Autodesk Inventor part; units mm, degrees
ref_plane "Work Plane1" through (0, 0, -12) normal (0, 0, 1) x (1, 0, 0)
ref_plane "YZ Plane" through (0, 0, 0) normal (1, 0, 0) x (0, 1, 0)
ref_plane "XZ Plane" through (0, 0, 0) normal (0, 1, 0) x (-1, 0, 0)
sketch "Sketch1" plane through (0, 0, 0) normal (0, 0, 1) x (1, 0, 0)
  line L0 (-199, 163) -> (199, 163)
  line L1 (199, 163) -> (199, -163)
  line L2 (199, -163) -> (-199, -163)
  line L3 (-199, -163) -> (-199, 163)
  line L4 (-199, 163) -> (199, -163) construction
  line L5 (199, 163) -> (-199, -163) construction
  point P0 (0, 0)
  dimension "d0" = 398
  dimension "d1" = 326
extrude "Extrusion1" add sketch "Sketch1" against normal blind 21
ref_plane "Work Plane1" through (0, 0, -12) normal (0, 0, 1) x (1, 0, 0)
sketch "Sketch2" plane through (0, 0, -12) normal (0, 0, 1) x (1, 0, 0)
  line L0 (-206, 163) -> (206, 163) construction
  line L1 (206, -170) -> (-206, -170) construction
  line L2 (-206, -170) -> (-206, 163) construction
  line L3 (-206, 163) -> (206, -170) construction
  line L4 (206, 163) -> (-206, -170) construction
  line L5 (-199, -163) -> (199, -163) construction
  line L6 (-199, 163) -> (-199, -163) construction
  line L7 (199, 163) -> (-199, 163) construction
  line L8 (-199, -163) -> (-199, 163)
  line L9 (199, 10.5) -> (206, 10.5)
  line L10 (206, 10.5) -> (206, -10.5)
  line L11 (206, -10.5) -> (199, -10.5)
  line L12 (199, -10.5) -> (199, 10.5)
  line L13 (199, 10.5) -> (206, -10.5) construction
  line L14 (206, 10.5) -> (199, -10.5) construction
  line L15 (206, -134.9) -> (199, -134.9)
  line L16 (199, -134.9) -> (199, -154.9)
  line L17 (199, -154.9) -> (206, -154.9)
  line L18 (206, -154.9) -> (206, -134.9)
  line L19 (199, -163) -> (-199, -163)
  line L20 (-8, -163) -> (8, -163)
  line L21 (8, -163) -> (8, -170)
  line L22 (8, -170) -> (-8, -170)
  line L23 (-8, -170) -> (-8, -163)
  line L24 (-139, -163) -> (-119, -163)
  line L25 (-119, -163) -> (-119, -170)
  line L26 (-119, -170) -> (-139, -170)
  line L27 (-139, -170) -> (-139, -163)
  line L28 (119, -163) -> (139, -163)
  line L29 (139, -163) -> (139, -170)
  line L30 (139, -170) -> (119, -170)
  line L31 (119, -170) -> (119, -163)
  line L32 (206, 163) -> (206, -170) construction
  line L33 (199, -163) -> (199, 163)
  line L34 (-288.4, 0) -> (288.4, 0)
  line L35 (0, 229.6) -> (0, -236.6)
  line L36 (206, 134.9) -> (199, 134.9)
  line L37 (199, 134.9) -> (199, 154.9)
  line L38 (199, 154.9) -> (206, 154.9)
  line L39 (206, 154.9) -> (206, 134.9)
  line L40 (-199, 10.5) -> (-206, 10.5)
  line L41 (-206, 10.5) -> (-206, -10.5)
  line L42 (-206, -10.5) -> (-199, -10.5)
  line L43 (-199, -10.5) -> (-199, 10.5)
  line L44 (-199, 10.5) -> (-206, -10.5) construction
  line L45 (-206, 10.5) -> (-199, -10.5) construction
  line L46 (-206, -134.9) -> (-199, -134.9)
  line L47 (-199, -134.9) -> (-199, -154.9)
  line L48 (-199, -154.9) -> (-206, -154.9)
  line L49 (-206, -154.9) -> (-206, -134.9)
  line L50 (-199, 134.9) -> (-199, 154.9)
  line L51 (-206, 134.9) -> (-199, 134.9)
  line L52 (-206, 154.9) -> (-206, 134.9)
  line L53 (-199, 154.9) -> (-206, 154.9)
  point P0 (0, 0)
  point P1 (0, -3.5)
  point P2 (202.5, 0)
  point P3 (202.5, 0)
  point P4 (-202.5, 0)
  point P5 (-202.5, 0)
  point P6 (0, -170)
  dimension "d6" = 7
  dimension "d7" = 7
  dimension "d8" = 0
  dimension "d9" = 21
  dimension "d10" = 20
  dimension "d11" = 124.4
  dimension "d12" = 7
  dimension "d13" = 16
  dimension "d14" = 111
  dimension "d15" = 20
  dimension "d16" = 111
  dimension "d17" = 20
extrude "Extrusion2" add sketch "Sketch2" against normal blind 1 contours L51 L52 L53 L8 | L33 L38 L39 L36 | L48 L49 L46 L8 | L19 L25 L26 L27 | L42 L41 L34 L8 | L19 L35 L22 L23 | L34 L41 L40 L8 | L19 L21 L22 L35 | L34 L10 L11 L12 | L12 L9 L10 L34 | L19 L29 L30 L31 | L15 L18 L17 L16
sketch "Sketch3" plane through (0, 0, -12) normal (0, 0, 1) x (1, 0, 0)
  line L0 (-119, -170) -> (-119, -163)
  line L1 (8, -170) -> (8, -163)
  line L2 (119, -163) -> (119, -170)
  point P0 (0, 0)
  point P1 (-202.5, 0)
  point P2 (202.5, 0)
  point P3 (129, -166.5)
  point P4 (0, -166.5)
  point P5 (-129, -166.5)
  point P6 (-119, -166.5)
  point P7 (8, -166.5)
  point P8 (119, -166.5)
hole "Hole1" at (-202.5, 0, -12) at (202.5, 0, -12) at (129, -166.5, -12) at (0, -166.5, -12) at (-129, -166.5, -12) direction (0, 0, -1) diameter 4 end through all
sketch "Sketch4" plane through (0, 0, -12) normal (0, 0, 1) x (1, 0, 0)
  line L0 (206, -134.9) -> (199, -134.9)
  point P0 (0, 0)
  point P1 (202.5, -139.9)
  dimension "d27" = 5
hole "Hole2" at (202.5, -139.9, -12) direction (0, 0, -1) diameter 4 end through all
sketch "Sketch5" plane through (0, 0, -12) normal (0, 0, 1) x (1, 0, 0)
  line L0 (199, -154.9) -> (206, -154.9)
  point P0 (0, 0)
  point P1 (202.5, -148.4)
  point P2 (202.5, -154.9)
  dimension "d35" = 6.5
hole "Hole3" at (202.5, -148.4, -12) direction (0, 0, -1) diameter 6 end through all
mirror "Mirror1" about plane through (0, 0, 0) normal (0, 1, 0) of "Hole2", "Hole3"
mirror "Mirror2" about plane through (0, 0, 0) normal (1, 0, 0) of "Hole2", "Hole3", "Mirror1"
sketch "Sketch6" plane through (0, 0, 0) normal (0, 0, 1) x (1, 0, 0)
  line L0 (-199, -163) -> (199, -163)
  line L1 (199, -163) -> (199, 163)
  line L2 (199, 163) -> (-199, 163)
  line L3 (-199, 163) -> (-199, -163)
  line L4 (-189.5, 153.5) -> (189.5, 153.5)
  line L5 (189.5, 153.5) -> (189.5, -153.5)
  line L6 (189.5, -153.5) -> (-189.5, -153.5)
  line L7 (-189.5, -153.5) -> (-189.5, 153.5)
  point P0 (0, 0)
  dimension "d43" = 9.5
extrude "Extrusion3" cut sketch "Sketch6" against normal blind 1 contours L4 L5 L6 L7
sketch "Sketch7" plane through (0, 0, -21) normal (0, 0, -1) x (-1, 0, 0)
  line L0 (32, 57) -> (127, 57)
  line L1 (127, 57) -> (127, -73)
  line L2 (127, -73) -> (32, -73)
  line L3 (32, -73) -> (32, 57)
  line L4 (199, -163) -> (199, 163)
  line L5 (-199, -163) -> (199, -163)
  point P0 (0, 0)
  dimension "d46" = 72
  dimension "d47" = 90
  dimension "d48" = 95
  dimension "d49" = 130
extrude "Extrusion4" add sketch "Sketch7" along normal blind 30
sketch "Sketch8" plane through (0, 0, -21) normal (0, 0, -1) x (-1, 0, 0)
  line L0 (-159, 91) -> (6, 91)
  line L1 (6, 91) -> (6, -71)
  line L2 (6, -71) -> (-159, -71)
  line L3 (-159, -71) -> (-159, 91)
  line L4 (-199, -163) -> (199, -163)
  line L5 (-199, 163) -> (-199, -163)
  point P0 (0, 0)
  dimension "d52" = 92
  dimension "d53" = 40
  dimension "d54" = 165
  dimension "d55" = 162
extrude "Extrusion5" add sketch "Sketch8" along normal blind 35
sketch "Sketch9" plane through (-6, -71, -21) normal (0, -1, 0) x (1, 0, 0)
  line L0 (0, 0) -> (165, 0)
  line L1 (0, 0) -> (0, -35)
  line L2 (165, -35) -> (0, -35)
  line L3 (165, 0) -> (165, -35)
  line L4 (165, 0) -> (165, -35)
  line L5 (165, -12) -> (135, -35)
  line L6 (165, -35) -> (0, -35)
  point P0 (6, 21)
  dimension "d58" = 23
  dimension "d59" = 30
extrude "Extrusion6" cut sketch "Sketch9" against normal through all contours L3 L2 L5
sketch "Sketch10" plane through (-127, -73, -21) normal (0, -1, 0) x (1, 0, 0)
  line L0 (0, 0) -> (95, 0)
  line L1 (0, 0) -> (0, -30)
  line L2 (95, -30) -> (0, -30)
  line L3 (95, 0) -> (95, -30)
  line L4 (95, -30) -> (0, -30)
  line L5 (12, -30) -> (6, -28)
  line L6 (6, -28) -> (0, -22)
  line L7 (0, 0) -> (0, -30)
  point P0 (127, 21)
  point P1 (0, -22)
  dimension "d62" = 6
  dimension "d63" = 12
  dimension "d64" = 2
  dimension "d65" = 8
extrude "Extrusion7" cut sketch "Sketch10" against normal through all contours L6 L5 L2 L1
properties part number "skærm"
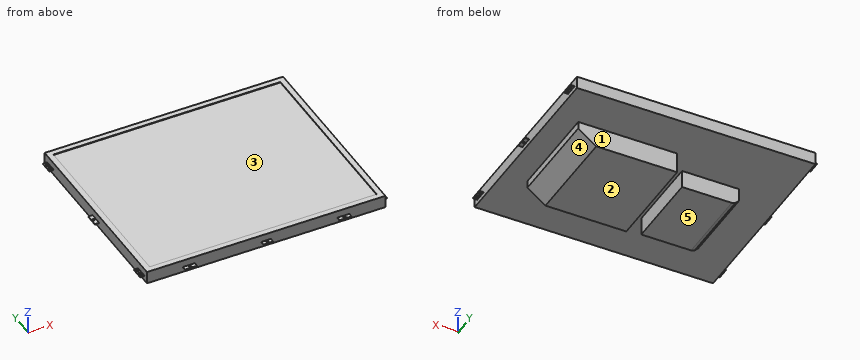
Work out the finished part from the listing and answer in its coordinate system (mm). Face numbers are marked on the shaded views. A direction names the side the tool comes from. Give positions to 0.01 mm unless a question says otherwise; leave off trailing zeros. Loops run counter-clockwise (first coordinate to the right, second up) from the corner with the lowest first, then second, coordinate; pieces in that order, holes last. Notation, with made-up numbers: (57, 1.5) -> (83, 1.5) arc R13 ccw to (83, 26.5) -> close; hole circle Ø6 at (60, -17). An arc over 180 degrees is marked (long way). Put each result on its own line as item: value. Start each with the question number.
Item 1: Each of these flat-tipped pins is pushed along its axis until it touches: P1, Ø4, axis at y = -42, z = -7, coming from the +X side; P2, Ø6.5, axis at x = -202.5, y = 139.9, coming from the +Z side; P3, Ø3, axis at x = 0, y = -166.5, coming from the -Z side; P4, Ø1.1, axis at x = 203.5, z = -12.5, coming from the +Y side. Where does it stop, or does it pass through?
Item 2: The part is cut by section A-A (z = -28). Give the vertices of the cut face in (x, y).
Item 3: The part is cut by section C-C (y = 20.5). Give the vertices of the cut face in (x, z), then the cut area to 3 significant figures.
Item 4: The part is cut by section B-B (x = 34.5). Give the vertices of the cut face in (y, z), then the cut area to 3 significant figures.
Item 5: Find the intervals of material crossed by L1, parallel to X at y = -166.5, z = -12.15; L2, parallel to X at y = -23.5, z = -30; L3, parallel to X at y = -139.9, z = -12.15, in increasing order. Write a range as [from, to].
Item 6: Which of the six approach directions +Z, -Z, +X, -X, +Y, -Y give full straight-line access (tool end or side, diameter ignored) to the marked faces 1 and 2?
Item 7: The mould has two halves that part along X. Classify the marked faces 3, 4 and 5: released by +X, released by -X, zero draft, split by the parting line, or undercut.
Answers below:
1. P1: x = 199
1. P2: z = -12
1. P3: through
1. P4: y = 154.9
2. outline: (-127, -73) -> (-32, -73) -> (-32, 57) -> (-127, 57) -> close; (-6, -71) -> (159, -71) -> (159, 91) -> (-6, 91) -> close
3. outline: (-199, -21) -> (-127, -21) -> (-127, -43) -> (-121, -49) -> (-115, -51) -> (-32, -51) -> (-32, -21) -> (-6, -21) -> (-6, -56) -> (129, -56) -> (159, -33) -> (159, -21) -> (199, -21) -> (199, 0) -> (189.5, 0) -> (189.5, -1) -> (-189.5, -1) -> (-189.5, 0) -> (-199, 0) -> close
3. area: 16,200 mm2
4. outline: (-163, -21) -> (-71, -21) -> (-71, -56) -> (91, -56) -> (91, -21) -> (163, -21) -> (163, 0) -> (153.5, 0) -> (153.5, -1) -> (-153.5, -1) -> (-153.5, 0) -> (-163, 0) -> close
4. area: 12,200 mm2
5. L1: [-139, -131], [-127, -119], [-8, -2], [2, 8], [119, 127], [131, 139]
5. L2: [-127, -32], [-6, 159]
5. L3: [-206, -204.5], [-200.5, 200.5], [204.5, 206]
6. face 1: -Z, +X, -X, +Y
6. face 2: -Z, +X, -X, +Y, -Y
7. face 3: undercut
7. face 4: released by +X
7. face 5: zero draft
